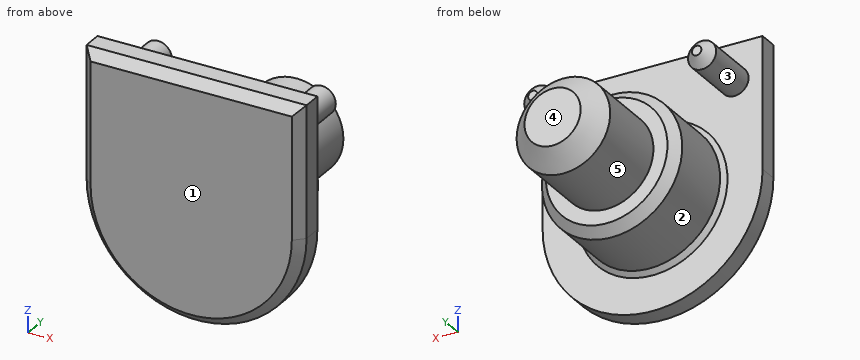
Autodesk Inventor part; units mm, degrees
ref_plane "YZ Plane" through (0, 0, 0) normal (1, 0, 0) x (0, 1, 0)
ref_plane "XZ Plane" through (0, 0, 0) normal (0, 1, 0) x (-1, 0, 0)
ref_plane "XY Plane" through (0, 0, 0) normal (0, 0, 1) x (1, 0, 0)
sketch "Boceto1" plane through (0, 0, 0) normal (0, 1, 0) x (-1, 0, 0)
  circle A0 centre (0, 0) radius 8
  circle A1 centre (8.75, 10) radius 1.5
  circle A2 centre (-8.75, 10) radius 1.5
  circle A3 centre (-8.75, 10) radius 1.5
  circle A4 centre (8.75, 10) radius 1.5
  line L0 (11.75, 10) -> (11.75, 14)
  line L1 (11.75, 14) -> (-8.75, 14)
  line L2 (-11.75, 10) -> (-11.75, 14)
  line L3 (-11.75, 14) -> (-8.75, 14)
  arc A5 (-11.75, 0) -> (11.75, 0) centre (0, 0) ccw
  line L4 (11.75, 0) -> (11.75, 10)
  line L5 (-11.75, 0) -> (-11.75, 10.3265)
extrude "Extrusión1" add sketch "Boceto1" along normal blind 3
sketch "Boceto2" plane through (0, 0, 0) normal (0, -1, 0) x (1, 0, 0)
  circle A0 centre (8.75, 10) radius 1.5
  circle A1 centre (8.75, 10) radius 1.5
  circle A2 centre (-8.75, 10) radius 1.5
  circle A3 centre (-8.75, 10) radius 1.5
  point P0 (0, 0)
extrude "Extrusión2" add sketch "Boceto2" against normal blind 10
sketch "Boceto3" plane through (0, 0, 0) normal (0, -1, 0) x (1, 0, 0)
  circle A0 centre (0, 0) radius 8
extrude "Extrusión3" add sketch "Boceto3" against normal blind 3.5
sketch "Boceto4" plane through (0, 3.5, 0) normal (0, 1, 0) x (1, 0, 0)
  circle A0 centre (0, 0) radius 7.5
  dimension "d16" = 15
extrude "Extrusión4" add sketch "Boceto4" along normal blind 8
sketch "Boceto5" plane through (0, 11.5, 0) normal (0, 1, 0) x (1, 0, 0)
  circle A0 centre (0, 0) radius 5
  dimension "d19" = 10
extrude "Extrusión5" add sketch "Boceto5" along normal blind 10
chamfer "Chaflán1" distance 0.5 angle 45 1 edges at (-8, 3.5, 0)
chamfer "Chaflán2" distance 1 angle 45 1 edges at (-7.5, 11.5, 0)
chamfer "Chaflán3" distance 2 angle 45 1 edges at (-5, 21.5, 0)
chamfer "Chaflán4" distance 1 angle 45 2 edges at (-10.25, 10, 10) (7.25, 10, 10)
chamfer "Chaflán5" distance 1 angle 45 4 edges at (0, 0, 14) (11.75, 0, 7) (0, 0, -11.75) (-11.75, 0, 7)
properties part number "soporte_brazo_art"
Here's how the part is built. I have some questions about the finished solid (model axes, mm). Face numbers are marked on the shaded views. A direction names the side the tool comes from. Coordinates: 2 decimals unless noted, no trailing zeros. Order: outer loops, then holes, each group sorted by start corner. A loop starts at its lowest first (then second) coordinate and runs counter-clockwise, first axis right, second up. Notation, with made-up numbers: M 18.25,34 L 26.25,34 A36 cw 26.25,70 Z; hole C -19.5,50.25 d7. An arc over 180 degrees is marked long. Answer as CSV lines item,"result".
Item 1: We'd pull the mould along X, two halves only. Please class the marked faces 1, 2 and 3: +X half, -X half, draft (parallel to the pull), parting line (faces both ways), or undercut.
Results found:
face 1,"draft"
face 2,"parting line"
face 3,"undercut"
Item 2: On a 3-axis mill with a long thin cutter (end or side, diameter ignored), from which of +Z, -Z, +X, -X, +Y, -Y can I reach the whole of each face in a straight line? I mean the marked faces 4 and 5. Say none if no direction works.
Results found:
face 4,"+Z, -Z, +X, -X, +Y"
face 5,"+Y"
Item 3: Imagine slicing it at C-C on y = 4. Write out the boundary of the cut face in (x, z).
Results found:
outline,"C -8.75,10 d3; C 0,0 d15; C 8.75,10 d3"
Item 4: For pin 1 (1.5 mm diameter, centred on x = -4.5, z = 2, fed in from -Y); pin 2 (1.5 mm diameter, centred on y = 16, z = 1.5, fed in from +X); pin 3 (12 mm diameter, centred on x = 8.5, y = 3.5, fed in from -Z); pin 4 (1 mm diameter, centred on x = 5, z = -9, fed in from +Y), each with a flat end and sliding along its axis, tell me the tip position at first contact or that it passes through.
Results found:
pin 1,"y = 0"
pin 2,"x = 4.94"
pin 3,"z = -11.48"
pin 4,"y = 3"
Item 5: Imagine slicing it at D-D on y = 18.5. Write out the boundary of the cut face in (x, z), plus the area to 3 significant figures.
Results found:
outline,"C 0,0 d10"
area,"78.5 mm2"
Item 6: Imagine slicing it at B-B on z = 10. Write out the boundary of the cut face in (x, y).
Results found:
outline,"M -11.75,1 L -10.75,0 L 10.75,0 L 11.75,1 L 11.75,3 L 10.25,3 L 10.25,9 L 9.25,10 L 8.25,10 L 7.25,9 L 7.25,3 L -7.25,3 L -7.25,9 L -8.25,10 L -9.25,10 L -10.25,9 L -10.25,3 L -11.75,3 Z"
Item 7: If I drill on line 1 (Y direction, x = -7.25, z = 12.25); line 2 (Z direction, x = 0.25, y = 2.5); line 3 (Y direction, x = 5.75, z = 0), over which ranges is the centre line in solid material (lowest first)?
Results found:
line 1,"0 to 3"
line 2,"-11.75 to 14"
line 3,"0 to 11.5"
